Here's how the part is built. I have some questions about the finished solid (model axes, mm). Face numbers are marked on the shaded views. Round coordinates to 2 decimals unless told otherwise and drop trailing zeros. Write each loop counter-clockwise with the first axis right and the second up, starting at its lowest first coordinate (ties: lowest second). Pieces come first, ordered by that corner, then holes. Notation, with made-up numbers: (-21, -28) - (6, -28) arc R21 ccw to (6, 3) - close; hole circle Ø2 at (5, -11). An arc over 180 degrees is marked (long way). Use one line per item in the form item = value. Start each with the question number.
1. I want a section at B-B, the plane y = 11.75. List the corners of the cut face in (x, z) for me, plus the area to 3 significant figures.
2. I want a section at C-C, the plane x = 18. List the corners of the cut face in (y, z) for me, plus the area to 3 significant figures.
3. If I drill on line 1 along X through (y, z) = (4.5, -95.25); line 2 along X through (y, z) = (7.5, -11.5); line 3 along Z through (x, y) = (87, 1), over which ranges is the centre line in solid material (lowest first)?
4. We'd pull the mould along Z, two halves only. Please class the marked faces 1 and 2: +Z half, -Z half, draft (parallel to the pull), parting line (faces both ways), or undercut.
5. Will these pins go through, and if not, where does the flat tip stop? pin 1 (3 mm diameter, centred on x = 59, z = -6.5, fed in from -Y); pin 2 (7 mm diameter, centred on x = 88, y = 5, fed in from -Z); pin 3 (4 mm diameter, centred on y = 4, z = -92, fed in from -X).
6. I want a section at A-A, the plane x = 30. List the corners of the cut face in (y, z) for me.
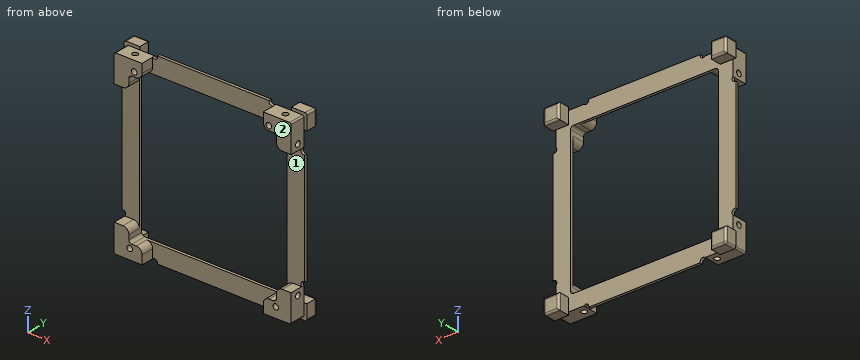
```python
from build123d import *

# Parameters (mm, degrees)
SKETCH1_W                         = 100
SKETCH1_H                         = 100
BOSS_EXTRUDE1_DEPTH               = 8.5
CUT_EXTRUDE1_DEPTH                = 142.676568281
SKETCH3_W                         = 8.5
SKETCH3_H                         = 8.5
BOSS_EXTRUDE2_DEPTH               = 6.5
TAP_DRILL_FOR_4_HELICOIL5_D       = 3.048
TAP_DRILL_FOR_4_HELICOIL5_DEPTH   = 5.69
TAP_DRILL_FOR_4_HELICOIL5_TIP     = 0.915711583
TAP_DRILL_FOR_4_HELICOIL5_4_D     = 3.048
TAP_DRILL_FOR_4_HELICOIL5_4_DEPTH = 5.69
TAP_DRILL_FOR_4_HELICOIL5_4_TIP   = 0.915711583
CUT_EXTRUDE2_DEPTH                = 7
CUT_EXTRUDE3_DEPTH                = 142.647449677
FILLET1_R                         = 1
FILLET2_R                         = 3.175
FILLET3_R                         = 0.79
TAP_DRILL_FOR_4_HELICOIL5_5_D     = 3.048
TAP_DRILL_FOR_4_HELICOIL5_5_DEPTH = 5.69
TAP_DRILL_FOR_4_HELICOIL5_5_TIP   = 0.915711583


with BuildPart() as part:
    # Sketch1 → Boss-Extrude1 (new body)
    with BuildSketch(Plane(origin=(0, 0, 0), x_dir=(1, 0, 0), z_dir=(0, 1, 0))):
        with Locations((50, 50)):
            Rectangle(SKETCH1_W, SKETCH1_H)
    extrude(amount=BOSS_EXTRUDE1_DEPTH)

    # Sketch2 → Cut-Extrude1 (cut, through all)
    with BuildSketch(Plane(origin=(0, 8.5, 0), x_dir=(1, 0, 0), z_dir=(0, 1, 0))):
        with BuildLine():
            Line((19.05, 100), (0, 100))
            Line((0, 100), (0, 83.590412453))
            Line((0, 83.590412453), (0, 80.95))
            Line((0, 80.95), (0, 80.554651577))
            ThreePointArc((0, 80.554651577), (1.825498063, 81.254538032), (1.5875, 83.19506403))
            Line((1.5875, 83.19506403), (1.5875, 98.4125))
            Line((1.5875, 98.4125), (16.80493597, 98.4125))
            ThreePointArc((16.80493597, 98.4125), (18.745461968, 98.174501937), (19.445348423, 100))
            Line((19.445348423, 100), (19.05, 100))
        make_face()
        with BuildLine():
            Line((80.95, 100), (80.554651577, 100))
            ThreePointArc((80.554651577, 100), (81.254538032, 98.174501937), (83.19506403, 98.4125))
            Line((83.19506403, 98.4125), (98.4125, 98.4125))
            Line((98.4125, 98.4125), (98.4125, 83.19506403))
            ThreePointArc((98.4125, 83.19506403), (98.174501937, 81.254538032), (100, 80.554651577))
            Line((100, 80.554651577), (100, 80.95))
            Line((100, 80.95), (100, 83.590412453))
            Line((100, 83.590412453), (100, 100))
            Line((100, 100), (80.95, 100))
        make_face()
        with BuildLine():
            Line((1.5875, 1.5875), (16.80493597, 1.5875))
            ThreePointArc((16.80493597, 1.5875), (18.745461968, 1.825498063), (19.445348423, 0))
            Line((19.445348423, 0), (19.05, 0))
            Line((19.05, 0), (0, 0))
            Line((0, 0), (0, 19.05))
            Line((0, 19.05), (0, 19.445348423))
            ThreePointArc((0, 19.445348423), (1.825498063, 18.745461968), (1.5875, 16.80493597))
            Line((1.5875, 16.80493597), (1.5875, 1.5875))
        make_face()
        with BuildLine():
            Line((98.4125, 1.5875), (83.19506403, 1.5875))
            ThreePointArc((83.19506403, 1.5875), (81.254538032, 1.825498063), (80.554651577, 0))
            Line((80.554651577, 0), (80.95, 0))
            Line((80.95, 0), (100, 0))
            Line((100, 0), (100, 19.05))
            Line((100, 19.05), (100, 19.445348423))
            ThreePointArc((100, 19.445348423), (98.174501937, 18.745461968), (98.4125, 16.80493597))
            Line((98.4125, 16.80493597), (98.4125, 1.5875))
        make_face()
    extrude(amount=-CUT_EXTRUDE1_DEPTH, mode=Mode.SUBTRACT)

    # Sketch3 → Boss-Extrude2 (add)
    with BuildSketch(Plane(origin=(0, 8.5, 0), x_dir=(1, 0, 0), z_dir=(0, 1, 0))):
        with Locations((4.25, 4.25)):
            Rectangle(SKETCH3_W, SKETCH3_H)
        with Locations((95.75, 4.25)):
            Rectangle(SKETCH3_W, SKETCH3_H)
        with Locations((95.75, 95.75)):
            Rectangle(SKETCH3_W, SKETCH3_H)
        with Locations((4.25, 95.75)):
            Rectangle(SKETCH3_W, SKETCH3_H)
    extrude(amount=BOSS_EXTRUDE2_DEPTH)

    # Tap Drill for _4 Helicoil5
    with Locations(Plane(origin=(0, 0, 0), x_dir=(-1, 0, 0), z_dir=(0, -1, 0))):
        with Locations((-86.195, 7.1375), (-90.005, 92.8625), (-12.535, 7.1375), (-9.995, 92.8625)):
            Hole(TAP_DRILL_FOR_4_HELICOIL5_D / 2, depth=TAP_DRILL_FOR_4_HELICOIL5_DEPTH)
            with Locations((0, 0, -(TAP_DRILL_FOR_4_HELICOIL5_DEPTH + TAP_DRILL_FOR_4_HELICOIL5_TIP / 2))):  # 118° drill point
                Cone(0, TAP_DRILL_FOR_4_HELICOIL5_D / 2, TAP_DRILL_FOR_4_HELICOIL5_TIP, mode=Mode.SUBTRACT)

    # Sketch18 → Tap Drill for _4 Helicoil5 2 (revolve, cut)
    with BuildSketch(Plane(origin=(1.5875, 4.5, -86.4125), x_dir=(0, 0, 1), z_dir=(0, 1, 0))):
        Polygon((0, 0), (0, 6.605711583), (1.524, 5.69), (1.524, 0), align=None)
    tap_drill_for_4_helicoil5_2 = revolve(axis=Axis((-4.7625, 4.5, -86.4125), (1, 0, 0)), mode=Mode.SUBTRACT)

    # Mirror1: Tap Drill for _4 Helicoil5 2 across plane
    add(tap_drill_for_4_helicoil5_2.mirror(Plane(origin=(0, 0, -50), x_dir=(1, 0, 0), z_dir=(0, 0, -1))), mode=Mode.SUBTRACT)

    # Mirror2: Tap Drill for _4 Helicoil5 2 across plane
    add(tap_drill_for_4_helicoil5_2.mirror(Plane.ZY.offset(-50)), mode=Mode.SUBTRACT)

    # Mirror2 copy 1 sketch → Mirror2 copy 1 (revolve, cut)
    with BuildSketch(Plane(origin=(98.4125, 4.5, -13.5875), x_dir=(0, 0, -1), z_dir=(0, 1, 0))):
        Polygon((0, 0), (0, 6.605711583), (1.524, 5.69), (1.524, 0), align=None)
    revolve(axis=Axis((104.7625, 4.5, -13.5875), (-1, 0, 0)), mode=Mode.SUBTRACT)

    # Sketch21 → Tap Drill for _4 Helicoil5 3 (revolve, cut)
    with BuildSketch(Plane(origin=(13.5875, 4.5, -98.4125), x_dir=(0, 1, 0), z_dir=(1, 0, 0))):
        Polygon((0, 0), (0, 6.605711583), (1.524, 5.69), (1.524, 0), align=None)
    tap_drill_for_4_helicoil5_3 = revolve(axis=Axis((13.5875, 4.5, -104.7625), (0, 0, 1)), mode=Mode.SUBTRACT)

    # Mirror3: Tap Drill for _4 Helicoil5 3 across plane
    add(tap_drill_for_4_helicoil5_3.mirror(Plane.ZY.offset(-50)), mode=Mode.SUBTRACT)

    # Tap Drill for _4 Helicoil5 4
    with Locations(Plane.XY.offset(-1.5875)):
        with Locations((91.6125, 4.5)):
            Hole(TAP_DRILL_FOR_4_HELICOIL5_4_D / 2, depth=TAP_DRILL_FOR_4_HELICOIL5_4_DEPTH)
            with Locations((0, 0, -(TAP_DRILL_FOR_4_HELICOIL5_4_DEPTH + TAP_DRILL_FOR_4_HELICOIL5_4_TIP / 2))):  # 118° drill point
                Cone(0, TAP_DRILL_FOR_4_HELICOIL5_4_D / 2, TAP_DRILL_FOR_4_HELICOIL5_4_TIP, mode=Mode.SUBTRACT)

    # Sketch22 → Cut-Extrude2 (cut)
    with BuildSketch(Plane.XZ):
        with BuildLine():
            Line((83.19506403, -9.5875), (88.825, -9.5875))
            ThreePointArc((88.825, -9.5875), (89.947532015, -10.052467985), (90.4125, -11.175))
            Line((90.4125, -11.175), (90.4125, -16.80493597))
            Line((90.4125, -16.80493597), (98.4125, -16.80493597))
            Line((98.4125, -16.80493597), (100, -16.80493597))
            Line((100, -16.80493597), (100, -83.19506403))
            Line((100, -83.19506403), (98.4125, -83.19506403))
            Line((98.4125, -83.19506403), (90.4125, -83.19506403))
            Line((90.4125, -83.19506403), (90.4125, -88.825))
            ThreePointArc((90.4125, -88.825), (89.947532015, -89.947532015), (88.825, -90.4125))
            Line((88.825, -90.4125), (83.19506403, -90.4125))
            Line((83.19506403, -90.4125), (83.19506403, -98.4125))
            Line((83.19506403, -98.4125), (83.19506403, -100))
            Line((83.19506403, -100), (16.80493597, -100))
            Line((16.80493597, -100), (16.80493597, -98.4125))
            Line((16.80493597, -98.4125), (16.80493597, -90.4125))
            Line((16.80493597, -90.4125), (11.175, -90.4125))
            ThreePointArc((11.175, -90.4125), (10.052467985, -89.947532015), (9.5875, -88.825))
            Line((9.5875, -88.825), (9.5875, -83.19506403))
            Line((9.5875, -83.19506403), (1.5875, -83.19506403))
            Line((1.5875, -83.19506403), (0, -83.19506403))
            Line((0, -83.19506403), (0, -16.80493597))
            Line((0, -16.80493597), (1.5875, -16.80493597))
            Line((1.5875, -16.80493597), (9.5875, -16.80493597))
            Line((9.5875, -16.80493597), (9.5875, -11.175))
            ThreePointArc((9.5875, -11.175), (10.052467985, -10.052467985), (11.175, -9.5875))
            Line((11.175, -9.5875), (16.80493597, -9.5875))
            Line((16.80493597, -9.5875), (16.80493597, -1.5875))
            Line((16.80493597, -1.5875), (16.80493597, 0))
            Line((16.80493597, 0), (83.19506403, 0))
            Line((83.19506403, 0), (83.19506403, -1.5875))
            Line((83.19506403, -1.5875), (83.19506403, -9.5875))
        make_face()
    extrude(amount=-CUT_EXTRUDE2_DEPTH, mode=Mode.SUBTRACT)

    # Sketch23 → Cut-Extrude3 (cut, through all)
    with BuildSketch(Plane.XZ.offset(-7)):
        with BuildLine():
            Line((11.175, -90.4125), (88.825, -90.4125))
            ThreePointArc((88.825, -90.4125), (89.947532015, -89.947532015), (90.4125, -88.825))
            Line((90.4125, -88.825), (90.4125, -11.175))
            ThreePointArc((90.4125, -11.175), (89.947532015, -10.052467985), (88.825, -9.5875))
            Line((88.825, -9.5875), (11.175, -9.5875))
            ThreePointArc((11.175, -9.5875), (10.052467985, -10.052467985), (9.5875, -11.175))
            Line((9.5875, -11.175), (9.5875, -88.825))
            ThreePointArc((9.5875, -88.825), (10.052467985, -89.947532015), (11.175, -90.4125))
        make_face()
    extrude(amount=-CUT_EXTRUDE3_DEPTH, mode=Mode.SUBTRACT)

    # Fillet1
    fillet1_edges = [part.edges().sort_by_distance(p)[0] for p in [
        (0, 11.75, 0),
        (0, 15, -4.25),
        (4.25, 15, 0),
        (8.5, 15, -4.25),
        (4.25, 15, -8.5),
        (100, 11.75, 0),
        (100, 15, -4.25),
        (95.75, 15, -8.5),
        (91.5, 15, -4.25),
        (95.75, 15, 0),
        (100, 11.75, -100),
        (95.75, 15, -100),
        (91.5, 15, -95.75),
        (95.75, 15, -91.5),
        (100, 15, -95.75),
        (0, 11.75, -100),
        (0, 15, -95.75),
        (4.25, 15, -91.5),
        (8.5, 15, -95.75),
        (4.25, 15, -100),
    ]]
    fillet(fillet1_edges, radius=FILLET1_R)

    # Fillet2
    fillet2_edges = [part.edges().sort_by_distance(p)[0] for p in [
        (9.5875, 3.5, -83.19506403),
        (90.4125, 3.5, -16.80493597),
        (90.4125, 3.5, -83.19506403),
        (83.19506403, 3.5, -90.4125),
        (16.80493597, 3.5, -90.4125),
        (9.5875, 3.5, -16.80493597),
        (16.80493597, 3.5, -9.5875),
        (83.19506403, 3.5, -9.5875),
    ]]
    fillet(fillet2_edges, radius=FILLET2_R)

    # Fillet3
    fillet3_edges = [part.edges().sort_by_distance(p)[0] for p in [
        (98.4125, 4.25, -98.4125),
        (1.5875, 4.25, -1.5875),
        (98.4125, 4.25, -1.5875),
        (1.5875, 4.25, -98.4125),
    ]]
    fillet(fillet3_edges, radius=FILLET3_R)

    # Tap Drill for _4 Helicoil5 5
    with Locations(Plane.XY.offset(-1.5875)):
        with Locations((9.2475, 4.5)):
            Hole(TAP_DRILL_FOR_4_HELICOIL5_5_D / 2, depth=TAP_DRILL_FOR_4_HELICOIL5_5_DEPTH)
            with Locations((0, 0, -(TAP_DRILL_FOR_4_HELICOIL5_5_DEPTH + TAP_DRILL_FOR_4_HELICOIL5_5_TIP / 2))):  # 118° drill point
                Cone(0, TAP_DRILL_FOR_4_HELICOIL5_5_D / 2, TAP_DRILL_FOR_4_HELICOIL5_5_TIP, mode=Mode.SUBTRACT)


solid = part.part
```
Model answer:
q1.outline = (0, -99) arc R1 ccw to (1, -100) - (8.5, -100) - (8.5, -91.5) - (0, -91.5) - close; (0, -8.5) - (8.5, -8.5) - (8.5, 0) - (1, 0) arc R1 ccw to (0, -1) - close; (91.5, -100) - (99, -100) arc R1 ccw to (100, -99) - (100, -91.5) - (91.5, -91.5) - close; (91.5, -8.5) - (100, -8.5) - (100, -1) arc R1 ccw to (99, 0) - (91.5, 0) - close
q1.area = 288 mm2
q2.outline = (7, -97.95) - (8.5, -97.95) - (8.5, -90.41) - (7, -90.41) - close; (7, -9.59) - (8.5, -9.59) - (8.5, -2.05) - (7, -2.05) - close
q2.area = 22.6 mm2
q3.line_1 = 1.59 to 12.06, 15.11 to 16.8, 83.2 to 84.89, 87.94 to 98.41
q3.line_2 = 1.59 to 9.59, 90.41 to 98.41
q3.line_3 = -98.41 to -90.41, -9.59 to -8.43, -5.84 to -1.59
q4.face_1 = undercut
q4.face_2 = draft
q5.pin_1 = 7
q5.pin_2 = -98.41
q5.pin_3 = 1.59
q6.outline = (7, -100) - (8.5, -100) - (8.5, -90.41) - (7, -90.41) - close; (7, -9.59) - (8.5, -9.59) - (8.5, 0) - (7, 0) - close
